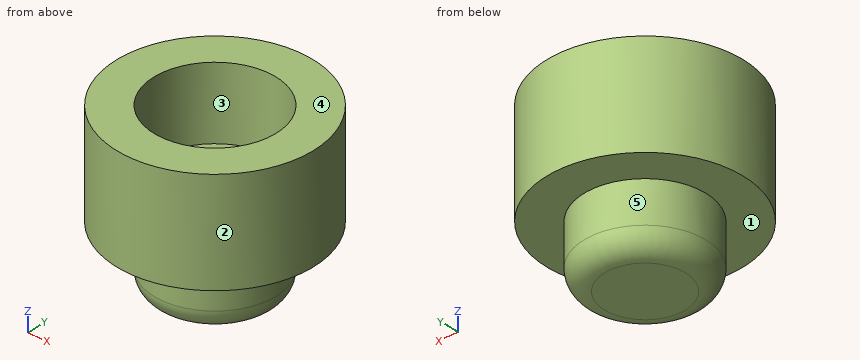
from build123d import *

# Parameters (mm, degrees)
F0_R          = 4.75
F0_R_2        = 2.95
F1_DEPTH      = 5
F2_DEPTH      = 3
F2_DEPTH_BACK = 1.5
F3_R          = 1


with BuildPart() as f1:
    # F0 (on Top) → F1 (new body)
    with BuildSketch(Plane.XY):
        Circle(F0_R)
        Circle(F0_R_2, mode=Mode.SUBTRACT)
    extrude(amount=F1_DEPTH)

    # F0 (on Top) → F2 (join, two sides)
    with BuildSketch(Plane.XY) as f2_sk:
        Circle(F0_R_2)
    extrude(amount=-F2_DEPTH)
    extrude(f2_sk.sketch, amount=F2_DEPTH_BACK)

    # F3
    f3_edges = [f1.edges().sort_by_distance(p)[0] for p in [
        (-2.95, 0, -3),
    ]]
    fillet(f3_edges, radius=F3_R)


solid = f1.part
Verification items for the finished model (mm, model axes). Face numbers are marked on the shaded views. A direction names the side the tool comes from. Coordinates: 2 decimals unless noted, no trailing zeros. Write each loop counter-clockwise with the first axis right and the second up, starting at its lowest first coordinate (ties: lowest second). Pieces come first, ordered by that corner, then holes. Notation, with made-up numbers: M 13.25,56 L 54.25,56 A7 cw 54.25,61 Z; hole C 85.5,62 d9. An arc over 180 degrees is marked long. Use a Markdown table: item, result.
Q1. Go/stop test with flat-tipped pins: P1, Ø3, axis at x = 0.5, y = 0, coming from the +Z side; P2, Ø1.5, axis at x = -1.5, z = 0, coming from the +Y side; P3, Ø5, axis at x = 2, y = -1, coming from the -Z side. Record where each tip stops, or that it passes through.
Reply:
| item | result |
|---|---|
| P1 | stops at z = 1.5 |
| P2 | stops at y = 4.69 |
| P3 | stops at z = -3 |
Q2. Sectioned sample at A-A, the plane x = 0. Record the boundary of the cut face in (y, z).
Reply:
| item | result |
|---|---|
| outline | M -4.75,0 L -2.95,0 L -2.95,-2 A1 ccw -1.95,-3 L 1.95,-3 A1 ccw 2.95,-2 L 2.95,0 L 4.75,0 L 4.75,5 L 2.95,5 L 2.95,1.5 L -2.95,1.5 L -2.95,5 L -4.75,5 Z |
Q3. Thickness scan on line 1 (Y direction, x = 0, z = 4.2); line 2 (Z direction, x = -2.5, y = 1.75); line 3 (Y direction, x = -2.5, z = 4.5). Record the ranges inside material, lowest first.
Reply:
| item | result |
|---|---|
| line 1 | y = -4.75 to -2.95, 2.95 to 4.75 |
| line 2 | z = 0 to 5 |
| line 3 | y = -4.04 to -1.57, 1.57 to 4.04 |
Q4. Sectioned sample at C-C, the plane z = 4.5. Record the boundary of the cut face in (x, y), plus the area to 3 significant figures.
Reply:
| item | result |
|---|---|
| outline | C 0,0 d9.5; hole C 0,0 d5.9 |
| area | 43.5 mm² |
Q5. Set-up check for the marked faces 4 and 5: record each of +Z, -Z, +X, -X, +Y, -Y from which the full face is reachable in a straight line by a thin tool's end or side.
Reply:
| item | result |
|---|---|
| face 4 | +Z, +X, -X, +Y, -Y |
| face 5 | -Z |
Q6. Sectioned sample at D-D, the plane y = 3.5. Record the boundary of the cut face in (x, z).
Reply:
| item | result |
|---|---|
| outline | M -3.21,0 L 3.21,0 L 3.21,5 L -3.21,5 Z |
Q7. Draft check along X on the marked faces 1, 2 and 3. Enter one of: +X half, -X half, draft (parallel to the pull), parting line (faces both ways), or undercut.
Reply:
| item | result |
|---|---|
| face 1 | draft |
| face 2 | parting line |
| face 3 | undercut |
